```python
from build123d import *

# Parameters (mm, degrees)
SKETCH3_W           = 21
SKETCH3_H           = 2
BOSS_EXTRUDE1_DEPTH = 12
CUT_EXTRUDE1_START  = -2
CUT_EXTRUDE1_DEPTH  = 8
CUT_EXTRUDE8_START  = -2
CUT_EXTRUDE8_DEPTH  = 36.336309405
CUT_EXTRUDE9_DEPTH  = 38.336309405
CUT_EXTRUDE11_DEPTH = 2
FILLET1_R           = 10


with BuildPart() as part:
    # Sketch3 → Boss-Extrude1 (new body)
    with BuildSketch(Plane.XY):
        with Locations((10.5, -1)):
            Rectangle(SKETCH3_W, SKETCH3_H)
        Polygon((13, 13), (0, 0), (17.494446501, 0), (25, 13), align=None)
        Polygon((25, 25), (13, 13), (25, 13), align=None)
    extrude(amount=BOSS_EXTRUDE1_DEPTH)

    # Sketch4 → Cut-Extrude1 (cut)
    with BuildSketch(Plane.XY.offset(12).offset(CUT_EXTRUDE1_START)):
        Polygon((25, 13), (20, 13), (3, 0), (17.494446501, 0), align=None)
    extrude(amount=-CUT_EXTRUDE1_DEPTH, mode=Mode.SUBTRACT)

    # Sketch7 → Cut-Extrude8 (cut, through all)
    with BuildSketch(Plane(origin=(0, 0, 0), x_dir=(0, 0, 1), z_dir=(-0.7071067811865485, 0.7071067811865466, 0)).offset(CUT_EXTRUDE8_START)):
        Polygon((6, 26.047596513), (6, 32.897596513), (4.022575328, 32.897596513), (2.045150656, 29.472596513), (4.022575328, 26.047596513), align=None)
        Polygon((7.977424672, 32.897596513), (6, 32.897596513), (6, 26.047596513), (7.977424672, 26.047596513), (9.954849344, 29.472596513), align=None)
    extrude(amount=-CUT_EXTRUDE8_DEPTH, mode=Mode.SUBTRACT)

    # Sketch8 → Cut-Extrude9 (cut, through all)
    with BuildSketch(Plane(origin=(0, 0, 0), x_dir=(0, 0, 1), z_dir=(-0.7071067811865485, 0.7071067811865466, 0))):
        with BuildLine():
            ThreePointArc((8, 29.355339059), (7.414213562, 30.769552622), (6, 31.355339059))
            Line((6, 31.355339059), (6, 27.355339059))
            ThreePointArc((6, 27.355339059), (7.414213562, 27.941125497), (8, 29.355339059))
        make_face()
        with BuildLine():
            Line((6, 27.355339059), (6, 31.355339059))
            ThreePointArc((6, 31.355339059), (4, 29.355339059), (6, 27.355339059))
        make_face()
    extrude(amount=-CUT_EXTRUDE9_DEPTH, mode=Mode.SUBTRACT)

    # Sketch9 → Cut-Extrude11 (cut)
    with BuildSketch(Plane(origin=(0, 0, 0), x_dir=(1, 0, 0), z_dir=(0, 1, 0))):
        with BuildLine():
            ThreePointArc((7.24722325, -2), (5.358620419, -4.950446591), (5.869726291, -8.416096101))
            Line((5.869726291, -8.416096101), (8.496224466, -6.96643844))
            ThreePointArc((8.496224466, -6.96643844), (9.28078481, -4.249001216), (11.998222034, -5.03356156))
            Line((11.998222034, -5.03356156), (14.62472021, -3.583903899))
            ThreePointArc((14.62472021, -3.583903899), (14.020027676, -2.718849781), (13.24722325, -2))
            Line((13.24722325, -2), (7.24722325, -2))
        make_face()
        with BuildLine():
            Line((8.496224466, -6.96643844), (5.869726291, -8.416096101))
            ThreePointArc((5.869726291, -8.416096101), (6.474418824, -9.281150219), (7.24722325, -10))
            Line((7.24722325, -10), (13.24722325, -10))
            ThreePointArc((13.24722325, -10), (14.719359205, -8.236067977), (15.24722325, -6))
            ThreePointArc((15.24722325, -6), (15.089097102, -4.752499458), (14.62472021, -3.583903899))
            Line((14.62472021, -3.583903899), (11.998222034, -5.03356156))
            ThreePointArc((11.998222034, -5.03356156), (12.183972791, -5.500999783), (12.24722325, -6))
            ThreePointArc((12.24722325, -6), (10.746223467, -7.936749541), (8.496224466, -6.96643844))
        make_face()
        with BuildLine():
            ThreePointArc((11.998222034, -5.03356156), (9.28078481, -4.249001216), (8.496224466, -6.96643844))
            Line((8.496224466, -6.96643844), (11.998222034, -5.03356156))
        make_face()
        with BuildLine():
            Line((11.998222034, -5.03356156), (8.496224466, -6.96643844))
            ThreePointArc((8.496224466, -6.96643844), (10.746223467, -7.936749541), (12.24722325, -6))
            ThreePointArc((12.24722325, -6), (12.183972791, -5.500999783), (11.998222034, -5.03356156))
        make_face()
        with BuildLine():
            ThreePointArc((13.24722325, -2), (10.24722325, -1), (7.24722325, -2))
            Line((7.24722325, -2), (13.24722325, -2))
        make_face()
        with BuildLine():
            Line((13.24722325, -10), (7.24722325, -10))
            ThreePointArc((7.24722325, -10), (10.24722325, -11), (13.24722325, -10))
        make_face()
    extrude(amount=CUT_EXTRUDE11_DEPTH, mode=Mode.SUBTRACT)

    # Sketch13 → CSK for M4 Flat Head Machine Screw1 (revolve, cut)
    with BuildSketch(Plane(origin=(10.24722325, 0, 6), x_dir=(0, 0, 1), z_dir=(1, 0, 0))):
        Polygon((0, 0), (0, 2), (2.15, 2), (2.15, 2.55), (4.7, 0), align=None)
    revolve(axis=Axis((10.24722325, 6.35, 6), (0, -1, 0)), mode=Mode.SUBTRACT)

    # Fillet1
    fillet1_edges = [part.edges().sort_by_distance(p)[0] for p in [
        (20, 13, 6),
    ]]
    fillet(fillet1_edges, radius=FILLET1_R)


solid = part.part
```
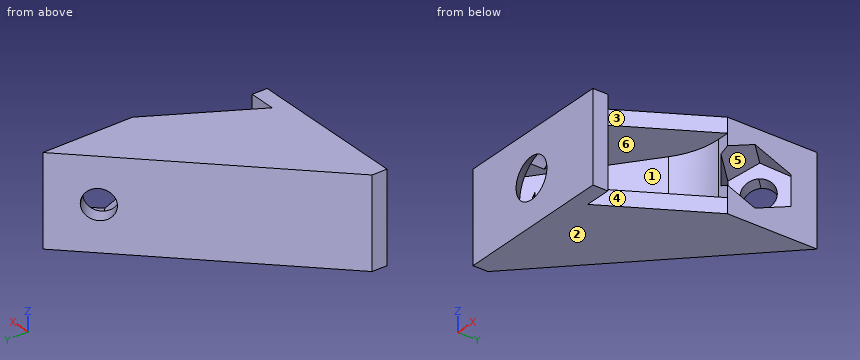
Could you check a few things on this model? Use its own coordinates, in mm. Face numbers are marked on the shaded views. A direction names the side the tool comes from. Round coordinates to 2 decimals unless told otherwise and drop trailing zeros. Order: outer loops, then holes, each group sorted by start corner. A loop starts at its lowest first (then second) coordinate and runs counter-clockwise, first axis right, second up. Notation, with made-up numbers: M 88.25,73.25 L 120.25,73.25 A24 cw 120.25,86.25 Z; hole C 44.25,80 d5. An arc over 180 degrees is marked long. One line per question, with ' | ' between items. Start each with the question number.
(1) Suppose I cut it at A-A on x = 4.5. List the corners of the cut face in (y, z) for me.
(2) Thinking about a two-plate mould opening in Z: for the marked faces 1, 2 and 3, which applies, +Z half, -Z half, draft (parallel to the pull), parting line (faces both ways), or undercut?
(3) Please list where these lines run through material, in increasing order: line 1 along Z through (x, y) = (11.5, 5.75); line 2 along Y through (x, z) = (14.75, 9); line 3 along Y through (x, z) = (18.75, 4.25).
(4) Suppose I cut it at D-D on y = 10.25. List the corners of the cut face in (x, z) for me, then the cut area to 3 significant figures.
(5) For P1, Ø1.3, axis at x = 24, z = 5.5, coming from the -Y side; P2, Ø6, axis at y = 5.5, z = 2.5, coming from the -X side; P3, Ø6, axis at y = 2.5, z = 9, coming from the +X side, each with a flat end and sliding along its axis, tell me the tip position at first contact or that it passes through.
(6) For the marked faces 4, 5 and 6, which set-ups out of +Z, -Z, +X, -X, +Y, -Y let a thin tool reach every point of the face, with its end or its side?
(7) Suppose I cut it at C-C on y = 14.5. List the corners of the cut face in (x, z) for me, then the cut area to 3 significant figures.
(8) Suppose I cut it at B-B on y = 0.5. List the corners of the cut face in (x, z) for me, then the cut area to 3 significant figures.
Geometry results:
1) outline: M -2,0 L 4.5,0 L 4.5,12 L -2,12 Z; hole M 0,2 L 1.15,2 L 1.15,10 L 0,10 Z
2) face 1: undercut | face 2: -Z half | face 3: draft
3) line 1: 0 to 2, 10 to 12 | line 2: -2 to 0, 8.99 to 14.75 | line 3: -2 to 0, 11.86 to 18.75
4) outline: M 10.25,0 L 23.41,0 L 23.41,2 L 16.4,2 L 16.4,10 L 23.41,10 L 23.41,12 L 10.25,12 Z | area: 102 mm²
5) P1: y = 13 | P2: x = 2.5 | P3: x = 21
6) face 4: +Z, -Z, +X | face 5: none | face 6: +X
7) outline: M 14.5,0 L 25,0 L 25,2.94 L 22.34,4.02 L 22.34,7.98 L 25,9.06 L 25,12 L 14.5,12 Z | area: 113 mm²
8) outline: M 0.5,0 L 17.78,0 L 17.78,2 L 13.25,2 A5 cw 7.25,2 L 3.65,2 L 3.65,10 L 7.25,10 A5 cw 13.25,10 L 17.78,10 L 17.78,12 L 0.5,12 Z | area: 86.2 mm²
